Here's how the part is built. I have some questions about the finished solid (model axes, mm). Coordinates: 2 decimals unless noted, no trailing zeros. Loops run counter-clockwise (first coordinate to the right, second up) from the corner with the lowest first, then second, coordinate; pieces in that order, holes last. Notation, with made-up numbers: (-39.5, 48) -> (-22.5, 48) arc R17 ccw to (-22.5, 73) -> close; hole circle Ø3 at (-36, 77). An arc over 180 degrees is marked (long way). Answer as a JSON object with one key per item and string values. Group by question number.
Q1. I want a section at C-C on z = -2.5. Write out the boundary of the cut face in (x, y).
Q2. I need wall thicknesses on line 1 (X direction, y = -1.5, z = -0.75); line 2 (X direction, y = -6.5, z = -0.75); line 3 (Y direction, x = 0, z = 2.4). Which ranges of each line are inside material? Lowest first, please.
Q3. I'm going to push flat-ended pins straight in: pin 1 (3 mm diameter, centred on x = 9.5, z = -2, fed in from +Y); pin 2 (2 mm diameter, centred on y = -12.5, z = -1.5, fed in from -X); pin 3 (4 mm diameter, centred on x = -12.5, z = 0, fed in from +Y). Where does each tip first touch, or does it pass through?
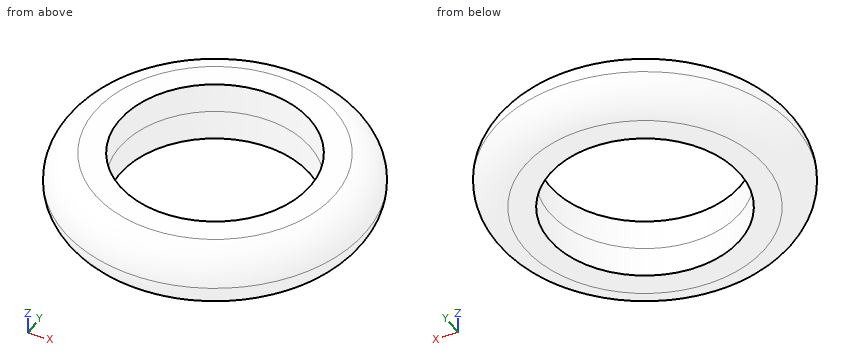
```python
from build123d import *

# Parameters (mm, degrees)
F0_R     = 17.3
F0_R_2   = 10.95
F1_DEPTH = 3.5
F2_DEPTH = 3.5
F3_R     = 3.49999
F4_R     = 3.49999


# Not quite as in the source:
# - a fillet or chamfer is up to 0.001 mm smaller than in the source, because OpenCascade refuses the exact size


with BuildPart() as f1:
    # F0 (on Top) → F1 (new body)
    with BuildSketch(Plane.XY):
        Circle(F0_R)
        Circle(F0_R_2, mode=Mode.SUBTRACT)
    extrude(amount=F1_DEPTH)

    # F2 (add): a face of the model
    f2_faces = [f1.faces().sort_by_distance(p)[0] for p in [
        (-16.8106821074, 0, 0),
    ]]
    extrude(f2_faces, amount=F2_DEPTH)

    # F3 (radius 3.5 in the source; OpenCascade refuses exactly that, so slightly less here)
    f3_edges = [f1.edges().sort_by_distance(p)[0] for p in [
        (-17.3, 0, 3.5),
    ]]
    fillet(f3_edges, radius=F3_R)

    # F4 (radius 3.5 in the source; OpenCascade refuses exactly that, so slightly less here)
    f4_edges = [f1.edges().sort_by_distance(p)[0] for p in [
        (-17.3, 0, -3.5),
    ]]
    fillet(f4_edges, radius=F4_R)


solid = f1.part
```
Result set:
{
 "1": {"outline": "circle Ø32.5 at (0, 0); hole circle Ø21.9 at (0, 0)"},
 "2": {"line 1": "x = -17.15 to -10.85, 10.85 to 17.15", "line 2": "x = -15.94 to -8.81, 8.81 to 15.94", "line 3": "y = -16.35 to -10.95, 10.95 to 16.35"},
 "3": {"pin 1": "stops at y = 14.98", "pin 2": "stops at x = -12.61", "pin 3": "stops at y = 13.75"}
}
